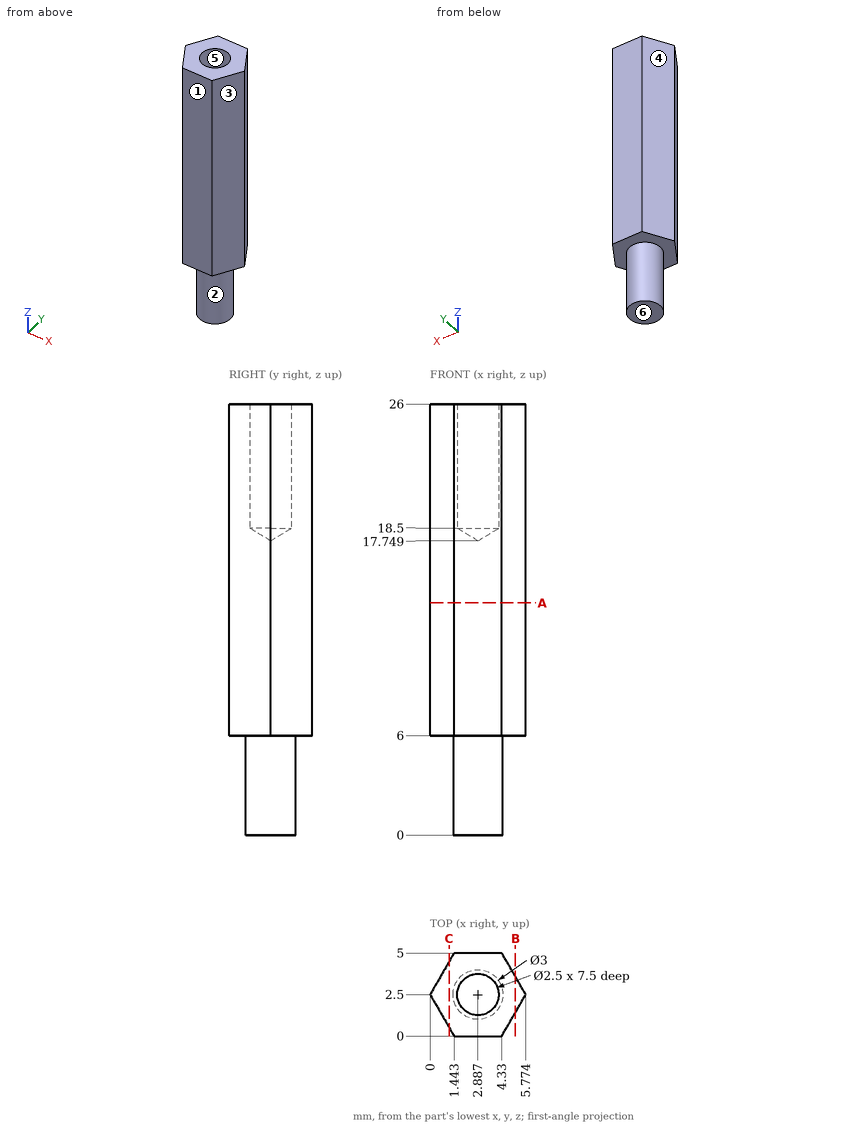
Drawing for the job (mm, zero at the part's lowest x, y, z). A direction names the side the tool comes from. Round coordinates to 2 decimals unless told otherwise and drop trailing zeros. Write each loop counter-clockwise with the first axis right and the second up, starting at its lowest first coordinate (ties: lowest second). Pieces come first, ordered by that corner, then holes. Notation, with made-up numbers: (17, -39) - (72, -39) arc R21 ccw to (72, -14) - close; hole circle Ø3 at (-23.75, -10.5). An arc over 180 degrees is marked (long way). Write item = value, one per line. Start each with the question number.
Q1. Band-saw the part on C-C (x = 1.15). Give the cut face in (y, z).
Q2. Band-saw the part on B-B (x = 5.15). Give the cut face in (y, z), then the cut area to 3 significant figures.
Q3. Drop flat-ended pins along their axis: pin 1 (2 mm diameter, centred on y = 3, z = 3.5, fed in from -X); pin 2 (2 mm diameter, centred on x = 2.89, y = 2.5, fed in from +Z). Give the stop position or say it passes through.
Q4. Mould opens along X. For the marked faces 3, 4, 5 and 6 say: pulls with the +X half, pulls with the -X half, needs draft (parallel to the pull), parting line crosses it, or undercut.
Q5. Band-saw the part on A-A (z = 14). Give the cut face in (x, y).
Q6. Probe L1, parallel to Z at x = 4.9, y = 3.9; L2, parallel to X at y = 2.8, z = 20.5 (1 decimal); L3, parallel to X at y = 2.55, z = 3 (1 decimal). List the from-to ranges inside material, lowest first. Write a range as from..to.
Q7. Which spindle directions (+Z, -Z, +X, -X, +Y, -Y) get a long thin tool onto all of the face, cutting with end or side? Do the marked faces 1 and 2. Say none if no direction does.
Answers below:
q1.outline = (0.51, 6) - (4.49, 6) - (4.49, 26) - (0.51, 26) - close
q2.outline = (1.42, 6) - (3.58, 6) - (3.58, 26) - (1.42, 26) - close
q2.area = 43.2 mm2
q3.pin_1 = 1.39
q3.pin_2 = 18.35
q4.face_3 = pulls with the +X half
q4.face_4 = pulls with the -X half
q4.face_5 = undercut
q4.face_6 = needs draft
q5.outline = (0, 2.5) - (1.44, 0) - (4.33, 0) - (5.77, 2.5) - (4.33, 5) - (1.44, 5) - close
q6.L1 = 6..26
q6.L2 = 0.2..1.7, 4.1..5.6
q6.L3 = 1.4..4.4
q7.face_1 = +Z, -Z, +X, -X, -Y
q7.face_2 = -Z
